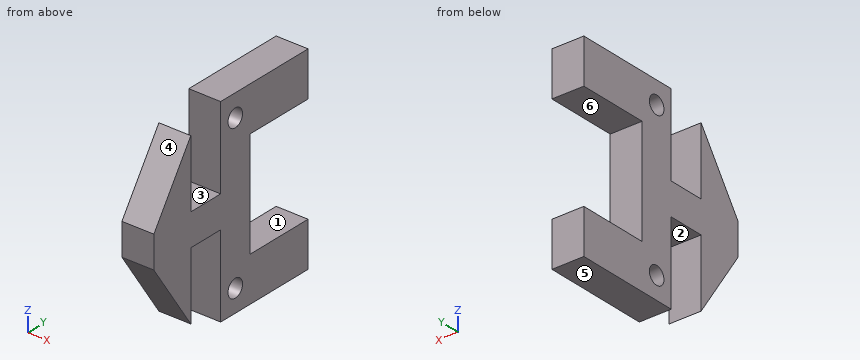
```python
from build123d import *

# Parameters (mm, degrees)
BOSS_EXTRUDE1_DEPTH = 3.5814
SKETCH7_R           = 1
CUT_EXTRUDE5_DEPTH  = 4.5814
BOSS_EXTRUDE3_DEPTH = 3.5814


with BuildPart() as part:
    # Sketch1 → Boss-Extrude1 (new body)
    with BuildSketch(Plane(origin=(0, 0, 0), x_dir=(0, 0, -1), z_dir=(1, 0, 0))):
        Polygon((-6, 6), (-6, -2), (6, -2), (6, 6), (11, 6), (11, -6), (-11, -6), (-11, 6), align=None)
    extrude(amount=BOSS_EXTRUDE1_DEPTH)

    # Sketch7 → Cut-Extrude5 (cut, through all)
    with BuildSketch(Plane(origin=(3.5814, 0, 0), x_dir=(0, 0, -1), z_dir=(1, 0, 0))):
        with Locations((-8.5, -4)):
            Circle(SKETCH7_R)
        with Locations((8.5, -4)):
            Circle(SKETCH7_R)
    extrude(amount=-CUT_EXTRUDE5_DEPTH, mode=Mode.SUBTRACT)

    # Sketch8 → Boss-Extrude3 (add)
    with BuildSketch(Plane(origin=(0, 0, 0), x_dir=(0, 0, -1), z_dir=(1, 0, 0))):
        Polygon((-1.7907, -10.1), (-9.398, -10.1), (-1.7907, -15.18), (1.7907, -15.18), (9.398, -10.1), (1.7907, -10.1), (1.7907, -6), (-1.7907, -6), align=None)
    extrude(amount=BOSS_EXTRUDE3_DEPTH)


solid = part.part
```
Input: part model. Units: mm. Frame: model coordinates. Face numbers are marked on the shaded views. A direction names the side the tool comes from. Give positions to 0.01 mm unless a question says otherwise; leave off trailing zeros. Order: outer loops, then holes, each group sorted by start corner. A loop starts at its lowest first (then second) coordinate and runs counter-clockwise, first axis right, second up. Notation, with made-up numbers: M -30,-39.75 L 18,-39.75 A22 ccw 18,-19.75 Z; hole C 46,50 d1. An arc over 180 degrees is marked long. Return JSON: item names as keys, results as strings.
Item 1: Access query for the marked faces 1, 2 and 3. Directions: +Z, -Z, +X, -X, +Y, -Y. A direction counts if a zero-diameter tool reaches every point of the face in a straight line with its end or side. Return the directions, or none.
Solutions:
{"face 1": "+X, -X, +Y", "face 2": "-Z, +X, -X", "face 3": "+Z, +X, -X"}
Item 2: Cut plane A-A (y = -4). Return loops of the section in (x, z).
Solutions:
{"outline": "M 0,-11 L 3.58,-11 L 3.58,-9.5 L 0,-9.5 Z; M 0,-7.5 L 3.58,-7.5 L 3.58,7.5 L 0,7.5 Z; M 0,9.5 L 3.58,9.5 L 3.58,11 L 0,11 Z"}
Item 3: First-contact query: P1, Ø2, axis at x = 2, z = 1.5, coming from the +Y side; P2, Ø1.1, axis at x = 2.5, y = -8, coming from the +Z side; P3, Ø1.1, axis at x = 2, z = -7, coming from the -Y side. Flat tips, straight axial feed; report the tip coordinate or a pass-through.
Solutions:
{"P1": "y = -2", "P2": "z = 1.79", "P3": "y = -12.07"}
Item 4: Cut plane C-C (z = -6.75). Return loops of the section in (x, y), then the cut area to 3 significant figures.
Solutions:
{"outline": "M 0,-11.87 L 3.58,-11.87 L 3.58,-10.1 L 0,-10.1 Z; M 0,-6 L 3.58,-6 L 3.58,6 L 0,6 Z", "area": "49.3 mm^2"}
Item 5: Ray query, probe 1 along Y at (x, z) = (0.5, -9); probe 2 along Y at (x, z) = (2.35, -8.5); probe 3 along Z at (x, y) = (2.6, -9.75). Return the intervals inside material, ascending.
Solutions:
{"probe 1": "-10.37 to -10.1, -6 to -4.87, -3.13 to 6", "probe 2": "-10.7 to -10.1, -6 to -5, -3 to 6", "probe 3": "-1.79 to 1.79"}
Item 6: Pull-direction query (Z, two-part tool) for the marked faces 4, 5 and 6; classes: +Z half, -Z half, draft (parallel to the pull), parting line (faces both ways), or undercut.
Solutions:
{"face 4": "+Z half", "face 5": "-Z half", "face 6": "undercut"}
Item 7: Cut plane D-D (z = 8.5). Return loops of the section in (x, y), then the cut area to 3 significant figures.
Solutions:
{"outline": "M 0,-10.7 L 3.58,-10.7 L 3.58,-10.1 L 0,-10.1 Z; M 0,-6 L 3.58,-6 L 3.58,-5 L 0,-5 Z; M 0,-3 L 3.58,-3 L 3.58,6 L 0,6 Z", "area": "38.0 mm^2"}
Item 8: Cut plane B-B (x = 0.9). Return loops of the section in (y, z), then the cut area to 3 significant figures.
Solutions:
{"outline": "M -15.18,-1.79 L -10.1,-9.4 L -10.1,-1.79 L -6,-1.79 L -6,-11 L 6,-11 L 6,-6 L -2,-6 L -2,6 L 6,6 L 6,11 L -6,11 L -6,1.79 L -10.1,1.79 L -10.1,9.4 L -15.18,1.79 Z; hole C -4,-8.5 d2; hole C -4,8.5 d2", "area": "233 mm^2"}
